Check sheet for the modelled part. Datum: model origin and axes. Units: mm. Face numbers are marked on the shaded views. Coordinates: 2 decimals unless noted, no trailing zeros. Write each loop counter-clockwise with the first axis right and the second up, starting at its lowest first coordinate (ties: lowest second). Pieces come first, ordered by that corner, then holes. Notation, with made-up numbers: (52.5, -37.5) -> (97.5, -37.5) arc R21 ccw to (97.5, -28.5) -> close; hole circle Ø2 at (-17, 59.5). An arc over 180 degrees is marked (long way). Put each result on its own line as item: value.
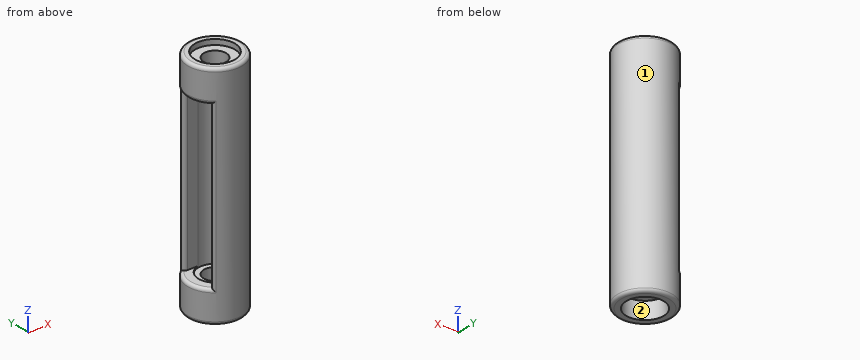
```python
from build123d import *

# Parameters (mm, degrees)
F0_R          = 5.1
F0_R_2        = 2.1
F1_DEPTH      = 42.6
F2_R          = 3.5
F3_DEPTH      = 3.2
F4_R          = 3.75
F5_DEPTH      = 1
F6_W          = 6
F6_H          = 30.6
F7_DEPTH      = 25
F9_START      = -2.5
F8_R          = 3.1
F9_DEPTH      = 31.5
F10_T1_DEPTH  = 30.6
F10_T10_ANGLE = 105.7758372511
F10_T16_ANGLE = 105.7758372511
F10_T23_DEPTH = 34.3907560857
F10_T27_ANGLE = 105.7758372511
F10_T34_ANGLE = 105.7758372511
F10_T38_DEPTH = 34.3907560857
F10_T45_DEPTH = 34.3907560857
F10_T49_ANGLE = 105.7758372511
F10_T56_DEPTH = 34.3907560857
F10_T60_ANGLE = 105.7758372511


# Not quite as in the source:
# - a fillet or chamfer that OpenCascade refuses, or shapes differently, is made with other operations: its cross-section is extruded or revolved along the edge and cut away or added


with BuildPart() as f1:
    # F0 (on Top) → F1 (new body)
    with BuildSketch(Plane.XY):
        Circle(F0_R)
        Circle(F0_R_2, mode=Mode.SUBTRACT)
    extrude(amount=F1_DEPTH)

    # F2 (on face) → F3 (cut)
    with BuildSketch(Plane(origin=(0, 0, 0), x_dir=(1, 0, 0), z_dir=(0, 0, -1))):
        Circle(F2_R)
    extrude(amount=-F3_DEPTH, mode=Mode.SUBTRACT)

    # F4 (on face) → F5 (cut)
    with BuildSketch(Plane.XY.offset(42.6)):
        Circle(F4_R)
    extrude(amount=-F5_DEPTH, mode=Mode.SUBTRACT)

    # F6 (on Right) → F7 (cut)
    with BuildSketch(Plane.YZ):
        with Locations((0, 21.3)):
            Rectangle(F6_W, F6_H)
    extrude(amount=-F7_DEPTH, mode=Mode.SUBTRACT)

    # F8 (on face) → F9 (cut)
    with BuildSketch(Plane(origin=(0, 0, 3.2), x_dir=(1, 0, 0), z_dir=(0, 0, -1)).offset(F9_START)):
        Circle(F8_R)
    extrude(amount=-F9_DEPTH, mode=Mode.SUBTRACT)

    # F10: fillet of radius 0.6 on 6 edges, made by hand

    # F10_s2 → F10_t1 (cut)
    with BuildSketch(Plane.XY.offset(6)):
        with BuildLine():
            ThreePointArc((-3.06, 4.08), (-3.2692099788, 3.4102633404), (-2.7, 3))
            Line((-2.7, 3), (-4.1243181255, 3))
            ThreePointArc((-4.1243181255, 3), (-3.6325207132, 3.5797755891), (-3.06, 4.08))
        make_face()
        with BuildLine():
            ThreePointArc((-3.06, -4.08), (-3.2692099788, -3.4102633404), (-2.7, -3))
            Line((-2.7, -3), (-4.1243181255, -3))
            ThreePointArc((-4.1243181255, -3), (-3.6325207132, -3.5797755891), (-3.06, -4.08))
        make_face()
    extrude(amount=F10_T1_DEPTH, mode=Mode.SUBTRACT)

    # F10_s3 → F10_t4 (revolve, cut)
    with BuildSketch(Plane.XZ):
        with BuildLine():
            ThreePointArc((5.1, 42), (4.9242640687, 42.4242640687), (4.5, 42.6))
            Line((4.5, 42.6), (5.1, 42.6))
            Line((5.1, 42.6), (5.1, 42))
        make_face()
    revolve(axis=Axis((0, 0, 42.6), (0, 0, 1)), mode=Mode.SUBTRACT)

    # F10_s5 → F10_t6 (revolve, cut)
    with BuildSketch(Plane.XZ):
        with BuildLine():
            ThreePointArc((5.1, 0.6), (4.9242640687, 0.1757359313), (4.5, 0))
            Line((4.5, 0), (5.1, 0))
            Line((5.1, 0), (5.1, 0.6))
        make_face()
    revolve(axis=Axis((0, 0, 0), (0, 0, 1)), mode=Mode.SUBTRACT)


with BuildPart() as f10_tool8:
    # F10_s9 → F10_t10 (revolve)
    with BuildSketch(Plane(origin=(0, 0, 0), x_dir=(0, 0, 1), z_dir=(0.7974567188, -0.6033761527, 0))):
        with BuildLine():
            ThreePointArc((5.4, 5.1), (5.8242640687, 4.9242640687), (6, 4.5))
            Line((6, 4.5), (6, 5.1))
            Line((6, 5.1), (5.4, 5.1))
        make_face()
    revolve(axis=Axis((0, 0, 6), (0, 0, -1)), revolution_arc=F10_T10_ANGLE)

    split(bisect_by=Plane.XZ.offset(3), keep=Keep.BOTTOM)

    split(bisect_by=Plane.XZ.offset(-3), keep=Keep.TOP)


with BuildPart() as f1_1:
    add(f1.part)

    # F10_t7: cut F10_tool8
    add(f10_tool8.part, mode=Mode.SUBTRACT)


with BuildPart() as f10_tool14:
    # F10_s15 → F10_t16 (revolve)
    with BuildSketch(Plane(origin=(0, 0, 0), x_dir=(0, 0, 1), z_dir=(0.7974567188, -0.6033761527, 0))):
        with BuildLine():
            ThreePointArc((37.2, 5.1), (36.7757359313, 4.9242640687), (36.6, 4.5))
            Line((36.6, 4.5), (36.6, 5.1))
            Line((36.6, 5.1), (37.2, 5.1))
        make_face()
    revolve(axis=Axis((0, 0, 36.6), (0, 0, -1)), revolution_arc=F10_T16_ANGLE)

    split(bisect_by=Plane.XZ.offset(3), keep=Keep.BOTTOM)

    split(bisect_by=Plane.XZ.offset(-3), keep=Keep.TOP)


with BuildPart() as f1_2:
    add(f1_1.part)

    # F10_t13: cut F10_tool14
    add(f10_tool14.part, mode=Mode.SUBTRACT)


with BuildPart() as f10_tool21:
    # F10_s22 → F10_t23 (new body)
    with BuildSketch(Plane.XY.offset(36.6)):
        with BuildLine():
            ThreePointArc((-3.06, -4.08), (-3.2692099788, -3.4102633404), (-2.7, -3))
            Line((-2.7, -3), (-4.1243181255, -3))
            ThreePointArc((-4.1243181255, -3), (-3.6325207132, -3.5797755891), (-3.06, -4.08))
        make_face()
    extrude(amount=-F10_T23_DEPTH)

    split(bisect_by=Plane.XY.offset(6), keep=Keep.BOTTOM)


with BuildPart() as f10_tool25:
    # F10_s26 → F10_t27 (revolve)
    with BuildSketch(Plane(origin=(0, 0, 0), x_dir=(0, 0, 1), z_dir=(0.7974567188, -0.6033761527, 0))):
        with BuildLine():
            ThreePointArc((5.4, 5.1), (5.8242640687, 4.9242640687), (6, 4.5))
            Line((6, 4.5), (6, 5.1))
            Line((6, 5.1), (5.4, 5.1))
        make_face()
    revolve(axis=Axis((0, 0, 6), (0, 0, -1)), revolution_arc=F10_T27_ANGLE)

    split(bisect_by=Plane.XZ.offset(3), keep=Keep.TOP)


with BuildPart() as f10_tool21_1:
    add(f10_tool21.part)

    # F10_t29: intersect F10_tool25
    add(f10_tool25.part, mode=Mode.INTERSECT)


with BuildPart() as f1_3:
    add(f1_2.part)

    # F10_t19: cut F10_tool21
    add(f10_tool21_1.part, mode=Mode.SUBTRACT)


with BuildPart() as f10_tool32:
    # F10_s33 → F10_t34 (revolve)
    with BuildSketch(Plane(origin=(0, 0, 0), x_dir=(0, 0, 1), z_dir=(0.7974567188, -0.6033761527, 0))):
        with BuildLine():
            ThreePointArc((5.4, 5.1), (5.8242640687, 4.9242640687), (6, 4.5))
            Line((6, 4.5), (6, 5.1))
            Line((6, 5.1), (5.4, 5.1))
        make_face()
    revolve(axis=Axis((0, 0, 6), (0, 0, -1)), revolution_arc=F10_T34_ANGLE)

    split(bisect_by=Plane.XZ.offset(-3), keep=Keep.BOTTOM)


with BuildPart() as f10_tool36:
    # F10_s37 → F10_t38 (new body)
    with BuildSketch(Plane.XY.offset(36.6)):
        with BuildLine():
            ThreePointArc((-3.06, 4.08), (-3.2692099788, 3.4102633404), (-2.7, 3))
            Line((-2.7, 3), (-4.1243181255, 3))
            ThreePointArc((-4.1243181255, 3), (-3.6325207132, 3.5797755891), (-3.06, 4.08))
        make_face()
    extrude(amount=-F10_T38_DEPTH)

    split(bisect_by=Plane.XY.offset(6), keep=Keep.BOTTOM)


with BuildPart() as f10_tool32_1:
    add(f10_tool32.part)

    # F10_t40: intersect F10_tool36
    add(f10_tool36.part, mode=Mode.INTERSECT)


with BuildPart() as f1_4:
    add(f1_3.part)

    # F10_t30: cut F10_tool32
    add(f10_tool32_1.part, mode=Mode.SUBTRACT)


with BuildPart() as f10_tool43:
    # F10_s44 → F10_t45 (new body)
    with BuildSketch(Plane.XY.offset(40.3907560857)):
        with BuildLine():
            ThreePointArc((-3.06, 4.08), (-3.2692099788, 3.4102633404), (-2.7, 3))
            Line((-2.7, 3), (-4.1243181255, 3))
            ThreePointArc((-4.1243181255, 3), (-3.6325207132, 3.5797755891), (-3.06, 4.08))
        make_face()
    extrude(amount=-F10_T45_DEPTH)

    split(bisect_by=Plane.XY.offset(36.6), keep=Keep.TOP)


with BuildPart() as f10_tool47:
    # F10_s48 → F10_t49 (revolve)
    with BuildSketch(Plane(origin=(0, 0, 0), x_dir=(0, 0, 1), z_dir=(0.7974567188, -0.6033761527, 0))):
        with BuildLine():
            ThreePointArc((37.2, 5.1), (36.7757359313, 4.9242640687), (36.6, 4.5))
            Line((36.6, 4.5), (36.6, 5.1))
            Line((36.6, 5.1), (37.2, 5.1))
        make_face()
    revolve(axis=Axis((0, 0, 36.6), (0, 0, -1)), revolution_arc=F10_T49_ANGLE)

    split(bisect_by=Plane.XZ.offset(-3), keep=Keep.BOTTOM)


with BuildPart() as f10_tool43_1:
    add(f10_tool43.part)

    # F10_t51: intersect F10_tool47
    add(f10_tool47.part, mode=Mode.INTERSECT)


with BuildPart() as f1_5:
    add(f1_4.part)

    # F10_t41: cut F10_tool43
    add(f10_tool43_1.part, mode=Mode.SUBTRACT)


with BuildPart() as f10_tool54:
    # F10_s55 → F10_t56 (new body)
    with BuildSketch(Plane.XY.offset(40.3907560857)):
        with BuildLine():
            ThreePointArc((-3.06, -4.08), (-3.2692099788, -3.4102633404), (-2.7, -3))
            Line((-2.7, -3), (-4.1243181255, -3))
            ThreePointArc((-4.1243181255, -3), (-3.6325207132, -3.5797755891), (-3.06, -4.08))
        make_face()
    extrude(amount=-F10_T56_DEPTH)

    split(bisect_by=Plane.XY.offset(36.6), keep=Keep.TOP)


with BuildPart() as f10_tool58:
    # F10_s59 → F10_t60 (revolve)
    with BuildSketch(Plane(origin=(0, 0, 0), x_dir=(0, 0, 1), z_dir=(0.7974567188, -0.6033761527, 0))):
        with BuildLine():
            ThreePointArc((37.2, 5.1), (36.7757359313, 4.9242640687), (36.6, 4.5))
            Line((36.6, 4.5), (36.6, 5.1))
            Line((36.6, 5.1), (37.2, 5.1))
        make_face()
    revolve(axis=Axis((0, 0, 36.6), (0, 0, -1)), revolution_arc=F10_T60_ANGLE)

    split(bisect_by=Plane.XZ.offset(3), keep=Keep.TOP)


with BuildPart() as f10_tool54_1:
    add(f10_tool54.part)

    # F10_t62: intersect F10_tool58
    add(f10_tool58.part, mode=Mode.INTERSECT)


with BuildPart() as f1_6:
    add(f1_5.part)

    # F10_t52: cut F10_tool54
    add(f10_tool54_1.part, mode=Mode.SUBTRACT)


solid = f1_6.part
```
Q1. Cross-section at B-B (x = 0). Record the cut outline in (y, z).
Recorded:
outline: (-5.1, 0.6) arc R0.6 ccw to (-4.5, 0) -> (-3.5, 0) -> (-3.5, 3.2) -> (-2.1, 3.2) -> (-2.1, 5.7) -> (-3.1, 5.7) -> (-3.1, 37.2) -> (-2.1, 37.2) -> (-2.1, 41.6) -> (-3.75, 41.6) -> (-3.75, 42.6) -> (-4.5, 42.6) arc R0.6 ccw to (-5.1, 42) -> close; (2.1, 3.2) -> (3.5, 3.2) -> (3.5, 0) -> (4.5, 0) arc R0.6 ccw to (5.1, 0.6) -> (5.1, 42) arc R0.6 ccw to (4.5, 42.6) -> (3.75, 42.6) -> (3.75, 41.6) -> (2.1, 41.6) -> (2.1, 37.2) -> (3.1, 37.2) -> (3.1, 5.7) -> (2.1, 5.7) -> close
Q2. Cross-section at A-A (y = 0). State how many separate pieces and enclosed holes the cut face has, plus the area to 3 significant figures.
Recorded:
separate pieces: 3
enclosed holes: 0
area: 119 mm2
Q3. Depth check by flat-ended pin: P1, Ø5.5, axis at x = 0, y = 0, coming from the +Z side; P2, Ø5, axis at x = -2, z = 30, coming from the -Y side; P3, Ø2, axis at x = -2, z = 23, coming from the +Y side; P4, Ø4.5, axis at x = 0, y = 0, coming from the -Z side. Enter the tip coordinate at first touch or a pass-through.
Recorded:
P1: stops at z = 41.6
P2: stops at y = -5.1
P3: stops at y = 5
P4: stops at z = 3.2
Q4. Material ranges on line 1 along Z through (x, y) = (-2.25, 1.5); line 2 along Y through (x, z) = (0, 40.55); line 3 along Z through (x, y) = (-3, 1.5), recorded low to high.
Recorded:
line 1: z = 3.2 to 5.7, 37.2 to 41.6
line 2: y = -5.1 to -2.1, 2.1 to 5.1
line 3: z = 3.2 to 6, 36.6 to 41.6
Q5. Mould release check, pull along X, two halves, no side actions. Record for the marked faces 1 and 2: released by +X, released by -X, zero draft, split by the parting line, or undercut.
Recorded:
face 1: split by the parting line
face 2: undercut
Q6. Cross-section at C-C (z = 36). Record the cut outline in (x, y), plus the area to 3 significant figures.
Recorded:
outline: (-3.06, -4.08) arc R5.1 ccw (long way) to (-3.06, 4.08) arc R0.6 ccw to (-2.7, 3) -> (-0.78, 3) arc R3.1 cw (long way) to (-0.78, -3) -> (-2.7, -3) arc R0.6 ccw to start
area: 36.8 mm2
